```python
from build123d import *

# Parameters (mm, degrees)
BOSS_EXTRUDE1_DEPTH = 30
BOSS_EXTRUDE2_DEPTH = 60
HOLE1_D             = 31.5
CIRPATTERN2_COUNT   = 6
CUT_EXTRUDE1_DEPTH  = 184.575597507
CIRPATTERN3_COUNT   = 6


with BuildPart() as part:
    # Sketch1 → Boss-Extrude1 (new body)
    with BuildSketch(Plane(origin=(0, 0, 0), x_dir=(1, 0, 0), z_dir=(0, 1, 0))):
        Polygon((40, -69.282032303), (80, 0), (40, 69.282032303), (-40, 69.282032303), (-80, 0), (-40, -69.282032303), align=None)
    extrude(amount=BOSS_EXTRUDE1_DEPTH)

    # Sketch2 → Boss-Extrude2 (add)
    with BuildSketch(Plane(origin=(0, 30, 0), x_dir=(1, 0, 0), z_dir=(0, 1, 0))):
        Polygon((20, -34.641016151), (40, 0), (20, 34.641016151), (-20, 34.641016151), (-40, 0), (-20, -34.641016151), align=None)
    extrude(amount=BOSS_EXTRUDE2_DEPTH)

    # Hole1 (through all)
    with Locations(Plane.XY.offset(34.641016151)):
        with Locations((0, 60)):
            hole1 = Hole(HOLE1_D / 2)

    # CirPattern2: Hole1 ×6 about axis
    cirpattern2_axis = Axis((0, 90, 0), (0, 1, 0))
    for i in range(1, CIRPATTERN2_COUNT):
        add(hole1.rotate(cirpattern2_axis, i * 360 / CIRPATTERN2_COUNT), mode=Mode.SUBTRACT)

    # Sketch5 → Cut-Extrude1 (cut, symmetric)
    with BuildSketch(Plane.XY.offset(69.282032303)):
        with BuildLine():
            Line((-10, 23), (10, 23))
            ThreePointArc((10, 23), (18, 15), (10, 7))
            Line((10, 7), (-10, 7))
            ThreePointArc((-10, 7), (-18, 15), (-10, 23))
        make_face()
    cut_extrude1 = extrude(amount=CUT_EXTRUDE1_DEPTH, both=True, mode=Mode.SUBTRACT)

    # CirPattern3: Cut-Extrude1 ×6 about axis
    cirpattern3_axis = Axis((0, 90, 0), (0, 1, 0))
    for i in range(1, CIRPATTERN3_COUNT):
        add(cut_extrude1.rotate(cirpattern3_axis, i * 360 / CIRPATTERN3_COUNT), mode=Mode.SUBTRACT)


solid = part.part
```
Geometry check sheet. Reference: the model listing, model coordinates, mm. A direction names the side the tool comes from. Give positions to 0.01 mm unless a question says otherwise; leave off trailing zeros. Loops run counter-clockwise (first coordinate to the right, second up) from the corner with the lowest first, then second, coordinate; pieces in that order, holes last. Notation, with made-up numbers: M 30.25,-31 L 62.25,-31 A18 cw 62.25,-27 Z; hole C 33.5,32.25 d11. An arc over 180 degrees is marked long. Write item = value, one per line. Start each with the question number.
1. Draft check along X on faces 4 (the face through (51.81, 14.82, -9.13)), 5 (the face through (-1, 0, -1)), 6 (the face through (34.584, 46.247, -9.38)). Enter one of: +X half, -X half, draft (parallel to the pull), parting line (faces both ways), or undercut.
2. Thickness scan on probe 1 along Y at (x, z) = (0, 17); probe 2 along Y at (x, z) = (10, -26); probe 3 along Y at (x, z) = (-41, 25). Record the ranges inside material, lowest first.
3. Tool access check on faces 1 (the face through (-51.184, 14.824, -8.769)), 2 (the face through (-9, 46, 34.641)), 3 (the face through (-18, 15, -49)). Record the directions out of +Z, -Z, +X, -X, +Y, -Y that give a thin tool (end or side, any length) a straight path to the whole face; none if there is none.
4. Section check A-A, the plane z = -52.5. Enter the section's corners in (x, y).
5. Go/stop test with flat-tipped pins: P1, Ø5, axis at y = 63, z = 5.5, coming from the +X side; P2, Ø1, axis at y = 24.5, z = -18.5, coming from the -X side; P3, Ø5, axis at x = 28.5, y = 43.5, coming from the +Z side. Record where each tip stops, or that it passes through.
6. Section check D-D, the plane x = -26. Give the number of separate pieces and of enclosed holes in the cut face, plus the area to 3 significant figures.
7. Section check C-C, the plane y = 35. Enter the section's corners in (x, z), plus the area to 3 significant figures.
8. Section check B-B, the plane y = 15. Enter the section's corners in (x, z), plus the area to 3 significant figures.
Values follow:
q1.face_4 = undercut
q1.face_5 = draft
q1.face_6 = +X half
q2.probe_1 = 0 to 7, 23 to 44.25, 75.75 to 90
q2.probe_2 = 0 to 7, 23 to 47.83, 72.17 to 90
q2.probe_3 = 0 to 7, 23 to 30
q3.face_1 = none
q3.face_2 = +Z, +X, -X, +Y
q3.face_3 = +Z, -Z
q4.outline = M -49.69,0 L 49.69,0 L 49.69,30 L -49.69,30 Z; hole M -10,7 L 10,7 A8 ccw 10,23 L -10,23 A8 ccw Z
q5.P1 = 38.27
q5.P2 = -69.61
q5.P3 = 24.25
q6.separate_pieces = 2
q6.enclosed_holes = 1
q6.area = 4,610 mm^2
q7.outline = M -40,0 L -20,-34.64 L 20,-34.64 L 40,0 L 20,34.64 L -20,34.64 Z
q7.area = 4,160 mm^2
q8.outline = M -80,0 L -69,-19.05 L -36,0 L -69,19.05 Z; M -51,-50.23 L -40,-69.28 L -18,-69.28 L -18,-31.18 Z; M -51,50.23 L -18,31.18 L -18,69.28 L -40,69.28 Z; M 18,-69.28 L 40,-69.28 L 51,-50.23 L 18,-31.18 Z; M 18,31.18 L 51,50.23 L 40,69.28 L 18,69.28 Z; M 36,0 L 69,-19.05 L 80,0 L 69,19.05 Z
q8.area = 5,030 mm^2
